from build123d import *

# Parameters (mm, degrees)
SKETCH_1_R           = 3
EXTRUDE_1_DEPTH      = 3
SKETCH_2_R           = 1.600000000000003
EXTRUDE_2_DEPTH      = 3
SKETCH_13_R          = 1.5250000000000004
CUT_EXTRUDE_8_DEPTH  = 10
CUT_EXTRUDE_9_DEPTH  = 10
CUT_EXTRUDE_10_DEPTH = 10
FILLET_7_R           = 3
FILLET_8_R           = 1.5
SKETCH_18_R          = 2.0999999999999996
CUT_EXTRUDE_11_DEPTH = 3
FILLET_2_R           = 2
SKETCH_12_R          = 1.600000000000003
CUT_EXTRUDE_7_DEPTH  = 10


with BuildPart() as part:
    # 草图1 → 凸台-拉伸1 (new body)
    with BuildSketch(Plane.XY):
        with BuildLine():
            Line((-18.999999999999996, -40), (19.000000000000004, -39.99999999999999))
            Line((19.000000000000004, -39.99999999999999), (19.000000000000004, -28.999999999999993))
            Line((19.000000000000004, -28.999999999999993), (12.222376083061231, 2.619832606143564))
            ThreePointArc((12.222376083061231, 2.619832606143564), (-2.01e-15, 12.500000000000007), (-12.222376083061231, 2.619832606143561))
            Line((-12.222376083061231, 2.619832606143561), (-18.999999999999996, -28.999999999999996))
            Line((-18.999999999999996, -28.999999999999996), (-18.999999999999996, -40))
        make_face()
        Circle(SKETCH_1_R, mode=Mode.SUBTRACT)
    extrude(amount=EXTRUDE_1_DEPTH)

    # 草图2 → 凸台-拉伸2 (add)
    with BuildSketch(Plane.XY.offset(3)):
        Polygon((-18.999999999999996, -40), (19.000000000000004, -39.99999999999999), (19.00000000000001, -90), (-18.99999999999999, -90), align=None)
        with Locations((-12.499999999999991, -83.99999999999999)):
            Circle(SKETCH_2_R, mode=Mode.SUBTRACT)
        with Locations((12.50000000000001, -83.99999999999999)):
            Circle(SKETCH_2_R, mode=Mode.SUBTRACT)
    extrude(amount=-EXTRUDE_2_DEPTH)

    # 草图13 → 切除-拉伸8 (cut)
    with BuildSketch(Plane.XY.offset(3)):
        with Locations((-12.999999999999984, -52.99999999999999)):
            Circle(SKETCH_13_R)
        with Locations((-12.999999999999982, -73)):
            Circle(SKETCH_13_R)
        with Locations((13.000000000000014, -52.99999999999999)):
            Circle(SKETCH_13_R)
        with Locations((13.000000000000016, -73)):
            Circle(SKETCH_13_R)
    extrude(amount=-CUT_EXTRUDE_8_DEPTH, mode=Mode.SUBTRACT)

    # 草图14 → 切除-拉伸9 (cut)
    with BuildSketch(Plane.XY.offset(3)):
        Polygon((-5.649695133285826, -55.49999999999999), (1.066e-14, -59.84591933329679), (1.375e-14, -55.49999999999999), align=None)
        Polygon((1.375e-14, -55.49999999999999), (1.483e-14, -59.845919333296784), (5.649695133285826, -55.49999999999999), align=None)
        Polygon((-10.499999999999963, -58.07715758978017), (-10.499999999999963, -67.92284241021984), (-4.100304866714181, -63.00000000000001), align=None)
        Polygon((-3.55e-15, -66.15408066670322), (-5.649695133285805, -70.5), (5.64969513328581, -70.5), align=None)
        Polygon((10.500000000000018, -58.077157589780114), (4.100304866714181, -63), (10.500000000000021, -67.92284241021987), align=None)
        Polygon((9.81e-15, -39.569701478766), (1.144e-14, -46.176084263737856), (8.588297620463438, -46.176084263737856), align=None)
        Polygon((-8.591336539479556, -46.176084263737856), (1.066e-14, -46.176084263737856), (9.81e-15, -39.569701478766), (-0.00151945950806542, -39.56853266375978), align=None)
        Polygon((-11.501519459508062, -30.722378817605943), (-11.501519459508062, -44.62978970986978), (-2.4617023795365665, -37.676084263737856), align=None)
        Polygon((-8.591336539479554, -29.176084263737856), (-0.00151945950806187, -35.78363586371593), (8.88e-15, -35.78246704870972), (7.23e-15, -29.176084263737856), align=None)
        Polygon((7.23e-15, -29.176084263737856), (8.87e-15, -35.78246704870972), (8.588297620463424, -29.176084263737856), align=None)
        Polygon((2.45866346052045, -37.67608426373786), (11.498480540491945, -44.62978970986978), (11.498480540491938, -30.72237881760594), align=None)
    extrude(amount=-CUT_EXTRUDE_9_DEPTH, mode=Mode.SUBTRACT)

    # 草图16 → 切除-拉伸10 (cut)
    with BuildSketch(Plane.XY.offset(3)):
        Polygon((-11.001870235626251, -6.000000000000001), (-15.112211013138483, -25.176084263737856), (-1.9999999999999978, -25.176084263737852), (-2, -6), align=None)
        Polygon((15.112211013138486, -25.17608426373785), (2.000000000000002, -25.176084263737856), (2, -5.999999999999999), (11.001870235626251, -5.999999999999998), align=None)
    extrude(amount=-CUT_EXTRUDE_10_DEPTH, mode=Mode.SUBTRACT)

    # 圆角7
    fillet_7_edges = [part.edges().sort_by_distance(p)[0] for p in [
        (-2.66e-15, -66.15408066670322, 1.5),
        (-0.00151945950806276, -35.78363586371593, 1.5),
        (1.274e-14, -59.84591933329679, 1.5),
        (-15.112211013138483, -25.176084263737856, 1.5),
        (-11.001870235626251, -6.000000000000001, 1.5),
        (-2, -6, 1.5),
        (-1.9999999999999978, -25.176084263737852, 1.5),
        (15.112211013138486, -25.17608426373785, 1.5),
        (2.000000000000002, -25.176084263737856, 1.5),
        (2, -5.999999999999999, 1.5),
        (11.001870235626251, -5.999999999999998, 1.5),
        (-0.00151945950806276, -39.56853266375978, 1.5),
    ]]
    fillet(fillet_7_edges, radius=FILLET_7_R)

    # 圆角8
    fillet_8_edges = [part.edges().sort_by_distance(p)[0] for p in [
        (4.1003048667141835, -63, 1.5),
        (10.500000000000016, -58.077157589780114, 1.5),
        (10.500000000000018, -67.92284241021987, 1.5),
        (-10.499999999999963, -67.92284241021984, 1.5),
        (-10.499999999999963, -58.07715758978017, 1.5),
        (-4.10030486671418, -63.00000000000001, 1.5),
        (-5.649695133285805, -70.5, 1.5),
        (5.64969513328581, -70.5, 1.5),
        (2.4586634605204445, -37.67608426373786, 1.5),
        (11.498480540491936, -30.722378817605943, 1.5),
        (11.498480540491942, -44.62978970986978, 1.5),
        (-11.501519459508062, -44.62978970986978, 1.5),
        (-11.501519459508062, -30.722378817605943, 1.5),
        (-2.4617023795365665, -37.676084263737856, 1.5),
        (8.588297620463425, -29.176084263737856, 1.5),
        (-8.591336539479554, -29.176084263737856, 1.5),
        (-5.649695133285826, -55.49999999999999, 1.5),
        (5.649695133285826, -55.49999999999999, 1.5),
        (8.588297620463436, -46.17608426373785, 1.5),
        (-8.591336539479556, -46.176084263737856, 1.5),
    ]]
    fillet(fillet_8_edges, radius=FILLET_8_R)

    # 草图18 → 切除-拉伸11 (cut)
    with BuildSketch(Plane(origin=(0, 0, 0), x_dir=(-1, 0, 0), z_dir=(0, 0, -1))):
        with Locations((-1.561e-14, -63)):
            Circle(SKETCH_18_R)
    extrude(amount=-CUT_EXTRUDE_11_DEPTH, mode=Mode.SUBTRACT)

    # 圆角2
    fillet_2_edges = [part.edges().sort_by_distance(p)[0] for p in [
        (-18.99999999999999, -90, 1.5),
        (19.00000000000001, -90, 1.5),
    ]]
    fillet(fillet_2_edges, radius=FILLET_2_R)

    # 草图12 → 切除-拉伸7 (cut)
    with BuildSketch(Plane.XY.offset(3)):
        with Locations((-12.499999999999991, -63.999999999999986)):
            Circle(SKETCH_12_R)
        with Locations((12.50000000000001, -63.999999999999986)):
            Circle(SKETCH_12_R)
    extrude(amount=-CUT_EXTRUDE_7_DEPTH, mode=Mode.SUBTRACT)


solid = part.part
CAD build for the part. Positions are in the model's coordinates, mm. Coordinates: 2 decimals unless noted, no trailing zeros. Order: outer loops, then holes, each group sorted by start corner. A loop starts at its lowest first (then second) coordinate and runs counter-clockwise, first axis right, second up. Notation, with made-up numbers: (72, 68.5) -> (98, 68.5) arc R23 ccw to (98, 95.5) -> close; hole circle Ø4 at (5.5, 6). An arc over 180 degrees is marked (long way). Answer in a Markdown table with one row per item.
1) Mould opens along X. For faces 1 (the face through (5.6, -30.2, 1.5)), 2 (the face through (-19, -59, 2)) say: pulls with the +X half, pulls with the -X half, needs draft (parallel to the pull), parting line crosses it, or undercut.
Check values:
| item | result |
|---|---|
| face 1 | undercut |
| face 2 | pulls with the -X half |
2) Band-saw the part on A-A (y = -84). List the corners of the cut face in (x, z).
Check values:
| item | result |
|---|---|
| outline | (-19, 0) -> (-14.1, 0) -> (-14.1, 3) -> (-19, 3) -> close; (-10.9, 0) -> (10.9, 0) -> (10.9, 3) -> (-10.9, 3) -> close; (14.1, 0) -> (19, 0) -> (19, 3) -> (14.1, 3) -> close |
3) Flat gauge pins, fed straight in: P1, Ø2.5, axis at x = -13, y = -73, coming from the +Z side; P2, Ø0.9, axis at x = 7, z = 1.5, coming from the +Y side; P3, Ø1.5, axis at y = -28, z = 1.5, coming from the -X side; P4, Ø1.5, axis at x = -9.5, z = 1.5, coming from the +Y side. Where does each tip first touch, or does it go through?
Check values:
| item | result |
|---|---|
| P1 | through |
| P2 | y = 10.65 |
| P3 | x = -18.95 |
| P4 | y = 8.93 |
4) Band-saw the part on B-B (z = 1.8). Give the number of separate pieces and of enclosed holes in the cut face, and give its area (3 significant figures).
Check values:
| item | result |
|---|---|
| separate pieces | 1 |
| enclosed holes | 20 |
| area | 2,680 mm2 |
5) Drill centre lines: line 1 (X direction, y = -73, z = 1.4) (3 decimals); line 2 (X direction, y = -15.5, z = 1.8); line 3 (Y direction, x = 9.5, z = 2.4). Where is each one in solid material? Low to high.
Check values:
| item | result |
|---|---|
| line 1 | -19 to -14.525, -11.475 to 11.475, 14.525 to 19 |
| line 2 | -16.11 to -13.04, -2 to 2, 13.04 to 16.11 |
| line 3 | -90 to -66.29, -59.71 to -43, -32.35 to -25.18, -6.15 to 8.12 |
6) Band-saw the part on C-C (y = 0). List the corners of the cut face in (x, z).
Check values:
| item | result |
|---|---|
| outline | (-12.78, 0) -> (-3, 0) -> (-3, 3) -> (-12.78, 3) -> close; (3, 0) -> (12.78, 0) -> (12.78, 3) -> (3, 3) -> close |
7) Band-saw the part on D-D (y = -24). List the corners of the cut face in (x, z), and give its area (3 significant figures).
Check values:
| item | result |
|---|---|
| outline | (-17.93, 0) -> (-13.78, 0) -> (-13.78, 3) -> (-17.93, 3) -> close; (-2.62, 0) -> (2.62, 0) -> (2.62, 3) -> (-2.62, 3) -> close; (13.78, 0) -> (17.93, 0) -> (17.93, 3) -> (13.78, 3) -> close |
| area | 40.6 mm2 |
